from build123d import *

# Parameters (mm, degrees)
EXTRUDE1_DEPTH     = 500
SKETCH3_R          = 25
CUT_EXTRUDE1_DEPTH = 672.710252301


with BuildPart() as part:
    # Sketch1 → Extrude1 (new body)
    with BuildSketch(Plane.XY):
        with BuildLine():
            Line((-25, 447.529481132), (0, 447.529481132))
            Line((0, 447.529481132), (0, -52.470518868))
            Line((0, -52.470518868), (-25, -52.470518868))
            Line((-25, -52.470518868), (-25, 0))
            Line((-25, 0), (-25, 165.029481132))
            ThreePointArc((-25, 165.029481132), (-33.786796564, 186.242684568), (-55, 195.029481132))
            Line((-55, 195.029481132), (-55.199777542, 195.029481132))
            Line((-55.199777542, 195.029481132), (-55.199777542, 200.029481132))
            Line((-55.199777542, 200.029481132), (-55, 200.029481132))
            ThreePointArc((-55, 200.029481132), (-33.786796564, 208.816277696), (-25, 230.029481132))
            Line((-25, 230.029481132), (-25, 447.529481132))
        make_face()
    extrude(amount=EXTRUDE1_DEPTH)

    # Sketch3 → Cut-Extrude1 (cut, through all)
    with BuildSketch(Plane.ZY.offset(25)):
        with Locations((450, 22.529481132)):
            Circle(SKETCH3_R)
        with Locations((250, 22.529481132)):
            Circle(SKETCH3_R)
        with Locations((50, 22.529481132)):
            Circle(SKETCH3_R)
        with Locations((450, 372.529481132)):
            Circle(SKETCH3_R)
        with Locations((250, 372.529481132)):
            Circle(SKETCH3_R)
        with Locations((50, 372.529481132)):
            Circle(SKETCH3_R)
    extrude(amount=-CUT_EXTRUDE1_DEPTH, mode=Mode.SUBTRACT)


solid = part.part
CAD build for the part. Positions are in the model's coordinates, mm. A direction names the side the tool comes from. Coordinates: 2 decimals unless noted, no trailing zeros. Loops run counter-clockwise (first coordinate to the right, second up) from the corner with the lowest first, then second, coordinate; pieces in that order, holes last. Notation, with made-up numbers: (-24.75, 34) - (-18.75, 34) arc R36 ccw to (-18.75, 73) - close; hole circle Ø5 at (-11, -22). An arc over 180 degrees is marked (long way). Write item = value, one per line. Start each with the question number.
Q1. Cut at B-B, the plane y = 6.5. List the corners of the cut face in (x, z), then the cut area to 3 significant figures.
Q2. Cut at D-D, the plane x = -7. List the corners of the cut face in (y, z).
Q3. Pull direction Y, two halves, no side cores. Call faces 1 (the flat face through (-25, 337, 246)), 2 (the flat face through (-12, -52.471, 246)), 3 (the cylindrical face through (-12.675, 30.039, 473.846)), 4 (the cylindrical face through (-34.021, 208.584, 246.5)): pulls with the +Y half, pulls with the -Y half, needs draft (parallel to the pull), parting line crosses it, or undercut.
Q4. Drill centre lines: L1, parallel to Y at x = -12, z = 452; L2, parallel to Y at x = -8.25, z = 250; L3, parallel to Z at x = -14.5, y = 28. Where is each one in solid material? Low to high.
Q5. Cut at A-A, the plane z = 50. List the corners of the cut face in (x, y).
Q6. Cut at C-C, the plane z = 418. List the corners of the cut face in (x, y).
Q7. Which spindle directions (+Z, -Z, +X, -X, +Y, -Y) get a long thin tool onto all of the face, cutting with end or side? Do faces 5 (the flat face through (-15, 201, 500)), 6 (the flat face through (-25, 55, 246)). Say none if no direction does.
Computed:
q1.outline = (-25, 0) - (0, 0) - (0, 30.82) - (-25, 30.82) - close; (-25, 69.18) - (0, 69.18) - (0, 230.82) - (-25, 230.82) - close; (-25, 269.18) - (0, 269.18) - (0, 430.82) - (-25, 430.82) - close; (-25, 469.18) - (0, 469.18) - (0, 500) - (-25, 500) - close
q1.area = 9,620 mm²
q2.outline = (-52.47, 0) - (447.53, 0) - (447.53, 500) - (-52.47, 500) - close; hole circle Ø50 at (22.53, 50); hole circle Ø50 at (22.53, 250); hole circle Ø50 at (22.53, 450); hole circle Ø50 at (372.53, 50); hole circle Ø50 at (372.53, 250); hole circle Ø50 at (372.53, 450)
q3.face_1 = needs draft
q3.face_2 = pulls with the -Y half
q3.face_3 = undercut
q3.face_4 = pulls with the +Y half
q4.L1 = -52.47 to -2.39, 47.45 to 347.61, 397.45 to 447.53
q4.L2 = -52.47 to -2.47, 47.53 to 347.53, 397.53 to 447.53
q4.L3 = 0 to 25.61, 74.39 to 225.61, 274.39 to 425.61, 474.39 to 500
q5.outline = (-55.2, 195.03) - (-55, 195.03) arc R30 cw to (-25, 165.03) - (-25, 47.53) - (0, 47.53) - (0, 347.53) - (-25, 347.53) - (-25, 230.03) arc R30 cw to (-55, 200.03) - (-55.2, 200.03) - close; (-25, -52.47) - (0, -52.47) - (0, -2.47) - (-25, -2.47) - close; (-25, 397.53) - (0, 397.53) - (0, 447.53) - (-25, 447.53) - close
q6.outline = (-55.2, 195.03) - (-55, 195.03) arc R30 cw to (-25, 165.03) - (-25, -52.47) - (0, -52.47) - (0, 447.53) - (-25, 447.53) - (-25, 230.03) arc R30 cw to (-55, 200.03) - (-55.2, 200.03) - close
q7.face_5 = +Z, +X, -X, +Y, -Y
q7.face_6 = +Z, -Z, -X, -Y
